Source: three-view drawing plus pictorial views. Frame: mm from the lowest corner of the part. A direction names the side the tool comes from. Give positions to 0.01 mm unless a question says otherwise; leave off trailing zeros. Order: outer loops, then holes, each group sorted by start corner. A loop starts at its lowest first (then second) coordinate and runs counter-clockwise, first axis right, second up.
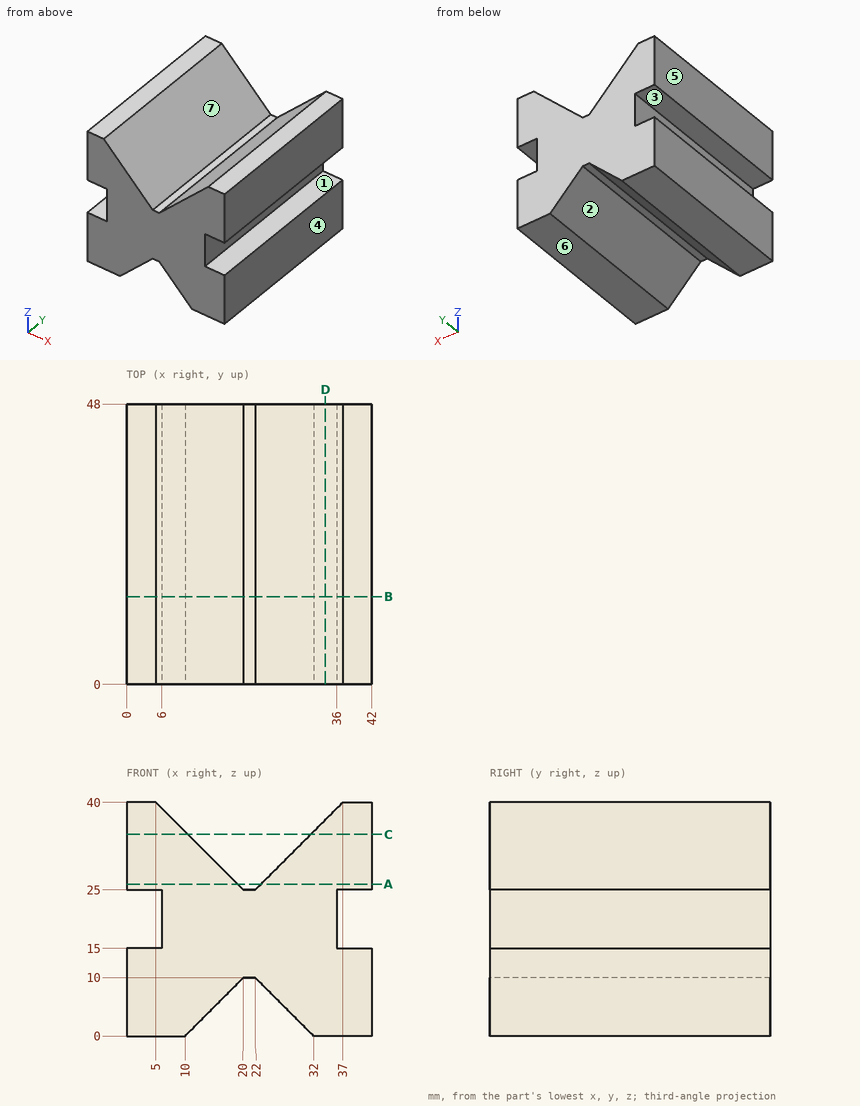
1) Section query C-C on z = 34.5. Output: boundary loops of the cut face in (x, y).
Checks:
outline: (0, 0) - (10.5, 0) - (10.5, 48) - (0, 48) - close; (31.5, 0) - (42, 0) - (42, 48) - (31.5, 48) - close
2) Section query A-A on z = 26. Output: boundary loops of the cut face in (x, y).
Checks:
outline: (0, 0) - (19, 0) - (19, 48) - (0, 48) - close; (23, 0) - (42, 0) - (42, 48) - (23, 48) - close
3) Section query D-D on x = 34. Output: boundary loops of the cut face in (y, z).
Checks:
outline: (0, 0) - (48, 0) - (48, 37) - (0, 37) - close
4) Reachability of the marked faces 1, 2 and 3 from +Z, -Z, +X, -X, +Y, -Y: full face, straight path, thin tool, end or side. Return the list, or none.
Checks:
face 1: +X, +Y, -Y
face 2: -Z, +Y, -Y
face 3: -X, +Y, -Y
5) Pull-direction query (X, two-part tool) for the marked faces 4, 5, 6 and 7; classes: +X half, -X half, draft (parallel to the pull), parting line (faces both ways), or undercut.
Checks:
face 4: +X half
face 5: -X half
face 6: draft
face 7: undercut
6) Ray query, L1, parallel to Z at x = 39.5, y = 27; L2, parallel to X at y = 32, z = 20; L3, parallel to X at y = 26.5, z = 3. Return the intervals inside material, ascending.
Checks:
L1: z = 0 to 15, 25 to 40
L2: x = 6 to 36
L3: x = 0 to 13, 29 to 42
7) Section query B-B on y = 15. Output: boundary loops of the cut face in (x, z).
Checks:
outline: (0, 0) - (10, 0) - (20, 10) - (22, 10) - (32, 0) - (42, 0) - (42, 15) - (36, 15) - (36, 25) - (42, 25) - (42, 40) - (37, 40) - (22, 25) - (20, 25) - (5, 40) - (0, 40) - (0, 25) - (6, 25) - (6, 15) - (0, 15) - close
8) First-contact query: pin 1 Ø5 at (x, y) = (40, 25.5) entering from -Z; pin 2 Ø1 at (x, y) = (21, 14) entering from -Z; pin 3 Ø8 at (y, z) = (34.5, 20) entering from +X; pin 4 Ø0.6 at (x, y) = (21, 26) entering from +Z. Flat tips, straight axial feed; report the tip coordinate or a pass-through.
Checks:
pin 1: stops at z = 0
pin 2: stops at z = 10
pin 3: stops at x = 36
pin 4: stops at z = 25
